For this review, take the finished solid that the model builds, in its own axes (mm). Face numbers are marked on the shaded views. Coordinates: 2 decimals unless noted, no trailing zeros. Order: outer loops, then holes, each group sorted by start corner. A loop starts at its lowest first (then second) coordinate and runs counter-clockwise, first axis right, second up. Notation, with made-up numbers: (68.25, 10.5) -> (103.25, 10.5) arc R13 ccw to (103.25, 25.5) -> close; hole circle Ø2 at (-31, 14). An arc over 180 degrees is marked (long way). Return JSON: item names as keys, results as strings. Group by question number.
Item 1: Take a section at A-A (z = 13). Write out the cut boundary in (x, y).
Item 2: Draft analysis for pull direction Y (two halves, no side actions). For the marked faces 1, 2, 3 and 4, state which applies: +Y half, -Y half, draft (parallel to the pull), parting line (faces both ways), or undercut.
Item 3: Insertion check: pin 1 (1.5 mm diameter, centred on x = -31.5, y = -3, fed in from +Z); pin 2 (1.5 mm diameter, centred on x = -27.5, y = -4.5, fed in from +Z); pin 3 (5 mm diameter, centred on x = -33.5, z = 15.5, fed in from +Y); pin 4 (1 mm diameter, centred on x = -27, y = -17.5, fed in from +Z). Each pin has a flat end and moves straight along its axis. Give the tip position at first contact, or say it passes through.
Item 4: Take a section at C-C (x = -29.25). Write out the cut boundary in (y, z), then the cut area to 3 significant figures.
Item 5: Take a section at D-D (y = -15.5). Write out the cut boundary in (x, z).
Item 6: For line 1 along Y through (x, z) = (-30, 15.85); line 2 along Y through (x, z) = (-31.75, 8.5); line 3 along X through (y, z) = (-7, 9.75), list the stretches that pass through material, from the lowest coordinate up.
Item 7: Take a section at B-B (y = -10). Write out the cut boundary in (x, z), then the cut area to 3 significant figures.
```python
from build123d import *

# Parameters (mm, degrees)
SKETCH009_R     = 6.45
PAD004_DEPTH    = 20
SKETCH010_R     = 1.6
POCKET005_DEPTH = 20
POCKET006_DEPTH = 10
SKETCH012_W     = 20
SKETCH012_H     = 6
POCKET007_DEPTH = 21


with BuildPart() as part:
    # Sketch009 → Pad004 (new body)
    with BuildSketch(Plane.XZ):
        with Locations((-30, 10)):
            Circle(SKETCH009_R)
    extrude(amount=PAD004_DEPTH)

    # Sketch010 → Pocket005 (cut)
    with BuildSketch(Plane.XY):
        with Locations((-30, -10)):
            Circle(SKETCH010_R)
    extrude(amount=POCKET005_DEPTH, mode=Mode.SUBTRACT)

    # Sketch011 → Pocket006 (cut)
    with BuildSketch(Plane.XY.offset(14)):
        Polygon((-27.25, -8.412287), (-30, -6.824574), (-32.75, -8.412287), (-32.75, -11.587713), (-30, -13.175426), (-27.25, -11.587713), align=None)
    extrude(amount=-POCKET006_DEPTH, mode=Mode.SUBTRACT)

    # Sketch012 → Pocket007 (cut)
    with BuildSketch(Plane.XZ):
        with Locations((-30.92, 3)):
            Rectangle(SKETCH012_W, SKETCH012_H)
    extrude(amount=POCKET007_DEPTH, mode=Mode.SUBTRACT)


solid = part.part
```
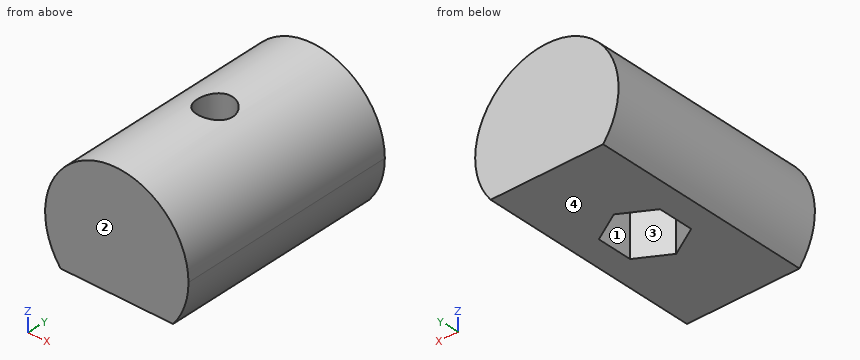
Findings below:
{
 "1": {"outline": "(-35.71, -20) -> (-24.29, -20) -> (-24.29, 0) -> (-35.71, 0) -> close; hole (-32.75, -11.59) -> (-30, -13.18) -> (-27.25, -11.59) -> (-27.25, -8.41) -> (-30, -6.82) -> (-32.75, -8.41) -> close"},
 "2": {"face 1": "undercut", "face 2": "-Y half", "face 3": "undercut", "face 4": "draft"},
 "3": {"pin 1": "stops at z = 16.41", "pin 2": "stops at z = 16.21", "pin 3": "stops at y = 0", "pin 4": "stops at z = 15.95"},
 "4": {"outline": "(-20, 6) -> (-12.74, 6) -> (-12.74, 14) -> (-11.41, 14) -> (-11.41, 16.41) -> (-20, 16.41) -> close; (-8.59, 14) -> (-7.26, 14) -> (-7.26, 6) -> (0, 6) -> (0, 16.41) -> (-8.59, 16.41) -> close", "area": "157 mm2"},
 "5": {"outline": "(-35.06, 6) -> (-24.94, 6) arc R6.45 ccw (long way) to start"},
 "6": {"line 1": "y = -20 to -11.6, -8.4 to 0", "line 2": "y = -20 to -12.17, -7.83 to 0", "line 3": "x = -36.45 to -30.3, -29.7 to -23.55"},
 "7": {"outline": "(-35.06, 6) -> (-32.75, 6) -> (-32.75, 14) -> (-31.6, 14) -> (-31.6, 16.25) arc R6.45 ccw to start; (-28.4, 14) -> (-27.25, 14) -> (-27.25, 6) -> (-24.94, 6) arc R6.45 ccw to (-28.4, 16.25) -> close", "area": "61.8 mm2"}
}
